Could you check a few things on this model? Use its own coordinates, in mm. Face numbers are marked on the shaded views. A direction names the side the tool comes from. Round coordinates to 2 decimals unless told otherwise and drop trailing zeros. Loops run counter-clockwise (first coordinate to the right, second up) from the corner with the lowest first, then second, coordinate; pieces in that order, holes last. Notation, with made-up numbers: (10, 7) -> (53, 7) arc R19 ccw to (53, 36) -> close; hole circle Ø1 at (-18, 30.5). An arc over 180 degrees is marked (long way). Write each question's results on one line, items separated by ' | '.
from build123d import *

# Parameters (mm, degrees)
EXTRUDE_1_DEPTH     = 5
CUT_EXTRUDE_1_DEPTH = 20
EXTRUDE_2_DEPTH     = 5


with BuildPart() as part:
    # 草图1 → 凸台-拉伸1 (new body)
    with BuildSketch(Plane(origin=(0, 0, 0), x_dir=(1, 0, 0), z_dir=(0, 1, 0))):
        Polygon((0, 20), (5.85, 20), (20, 5.85), (20, 0), (14.15, 0), (9.907359313, 0), (-11.819805153, -21.727164466), (-21.727164466, -11.819805153), (0, 9.907359313), align=None)
    extrude(amount=EXTRUDE_1_DEPTH)

    # 草图2 → 切除-拉伸1 (cut)
    with BuildSketch(Plane(origin=(4.953679656, 0, 4.953679656), x_dir=(0.7071067811865477, 0, -0.7071067811865475), z_dir=(0.7071067811865475, 0, 0.7071067811865477))):
        with BuildLine():
            Line((-23.721289706, 2), (-23.721289706, 5))
            Line((-23.721289706, 5), (7.005560954, 5))
            ThreePointArc((7.005560954, 5), (-8.284812198, 2.751778874), (-23.721289706, 2))
        make_face()
    extrude(amount=-CUT_EXTRUDE_1_DEPTH, mode=Mode.SUBTRACT)

    # 草图3 → 凸台-拉伸2 (add)
    with BuildSketch(Plane(origin=(0, 5, 0), x_dir=(1, 0, 0), z_dir=(0, 1, 0))):
        Polygon((0, 9.907359313), (0, 0), (9.907359313, 0), align=None)
    extrude(amount=-EXTRUDE_2_DEPTH)


solid = part.part
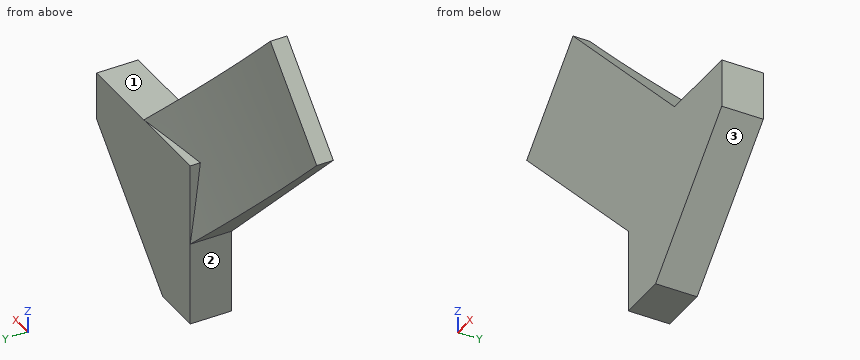
1) I need wall thicknesses on line 1 (Y direction, x = 1, z = 1); line 2 (Z direction, x = 1, y = 4.55); line 3 (Z direction, x = 4.5, y = 0.5). Which ranges of each line are inside material? Lowest first, please.
Model answer:
line 1: y = 0 to 3.78 | line 2: z = -20 to 0 | line 3: z = -20 to 5.41
2) I'm going to push flat-ended pins straight in: pin 1 (3 mm diameter, centred on y = 3.5, z = 9.5, fed in from +X); pin 2 (1.5 mm diameter, centred on x = -12, y = 2.5, fed in from -Z); pin 3 (10 mm diameter, centred on x = -14.5, z = 6.5, fed in from +Y). Where does each tip first touch, or does it pass through?
Model answer:
pin 1: stops at x = 1.87 | pin 2: stops at z = 1.34 | pin 3: stops at y = 2.61
3) I want a section at A-A, the plane y = 0.9. Write out the boundary of the cut face in (x, z), plus the area to 3 significant figures.
Model answer:
outline: (-21.73, 11.82) -> (0, -9.91) -> (0, -20) -> (5.85, -20) -> (20, -5.85) -> (20, 0) -> (9.91, 0) -> (-11.82, 21.73) -> close | area: 681 mm2
4) I want a section at B-B, the plane z = -17. Write out the boundary of the cut face in (x, y).
Model answer:
outline: (0, 0) -> (8.85, 0) -> (8.85, 5) -> (0, 5) -> close
5) I want a section at C-C, the plane z = -12.5. Write out the boundary of the cut face in (x, y).
Model answer:
outline: (0, 0) -> (13.35, 0) -> (13.35, 5) -> (0, 5) -> close
6) For the marked faces 1, 2 and 3, which set-ups out of +Z, -Z, +X, -X, +Y, -Y let a thin tool reach every point of the face, with its end or its side?
Model answer:
face 1: +Z, +X, +Y, -Y | face 2: -Z, -X, +Y, -Y | face 3: -Z, +X, +Y, -Y
